Geometry check sheet. Reference: the model listing, model coordinates, mm. Face numbers are marked on the shaded views. A direction names the side the tool comes from. Round coordinates to 2 decimals unless told otherwise and drop trailing zeros. Write each loop counter-clockwise with the first axis right and the second up, starting at its lowest first coordinate (ties: lowest second). Pieces come first, ordered by that corner, then holes. Notation, with made-up numbers: M -4.75,62 L 16.25,62 A29 ccw 16.25,100 Z; hole C 26,21 d2. An arc over 180 degrees is marked long. Answer in a Markdown table with one row per item. Add a question column.
from build123d import *

# Parameters (mm, degrees)
BOSS_EXTRUDE1_DEPTH      = 10
BOSS_EXTRUDE1_DEPTH_BACK = 0.01
SKETCH3_W                = 37
SKETCH3_H                = 40
CUT_EXTRUDE1_DEPTH       = 3
SKETCH5_W                = 37
SKETCH5_H                = 40
CUT_EXTRUDE3_DEPTH       = 3
SKETCH7_W                = 165
SKETCH7_H                = 54
CUT_EXTRUDE4_DEPTH       = 6
SKETCH9_W                = 19
SKETCH9_H                = 16
SKETCH9_W_2              = 13.23867097
SKETCH9_H_2              = 10.64338859
SKETCH9_W_3              = 14.8958404
SKETCH9_H_3              = 14.23867097
BOSS_EXTRUDE2_DEPTH      = 20.3
SKETCH15_W               = 20
SKETCH15_H               = 50
BOSS_EXTRUDE3_DEPTH      = 20.3
SKETCH16_W               = 7.597238681
SKETCH16_H               = 8
SKETCH16_W_2             = 10
SKETCH16_H_2             = 9.4
SKETCH16_W_3             = 8.7
SKETCH16_H_3             = 8.5
SKETCH16_W_4             = 9.4
SKETCH16_H_4             = 9.3
BOSS_EXTRUDE4_DEPTH      = 30
SKETCH17_R               = 2.55
SKETCH17_R_2             = 3.5
CUT_EXTRUDE17_DEPTH      = 263.98121496
SKETCH18_W               = 43.4
SKETCH18_H               = 43.4
CUT_EXTRUDE18_DEPTH      = 3
SKETCH20_R               = 5
SKETCH20_R_2             = 4
CUT_EXTRUDE20_DEPTH      = 263.98121496
SKETCH21_R               = 9
CUT_EXTRUDE21_DEPTH      = 20
SKETCH22_R               = 1.55
CUT_EXTRUDE23_DEPTH      = 263.007861374
SKETCH25_W               = 7.9
SKETCH25_H               = 58.5
BOSS_EXTRUDE5_DEPTH      = 4
SKETCH26_W               = 7.816347336
SKETCH26_H               = 2.399791276
CUT_EXTRUDE24_DEPTH      = 58.5


with BuildPart() as part:
    # Sketch1 → Boss-Extrude1 (new, two sides: drawn at the far end of the back side and taken through both)
    with BuildSketch(Plane.XY.offset(-BOSS_EXTRUDE1_DEPTH_BACK)):
        with BuildLine():
            Line((0, 0), (0, -26))
            Line((0, -26), (60, -26))
            Line((60, -26), (60, -41))
            Line((60, -41), (33.129942315, -67.870057685))
            Line((33.129942315, -67.870057685), (-55.850057685, -67.870057685))
            ThreePointArc((-55.850057685, -67.870057685), (-169.745893523, -93.14097487), (-240, 0))
            ThreePointArc((-240, 0), (-169.745893523, 93.14097487), (-55.850057685, 67.870057685))
            Line((-55.850057685, 67.870057685), (33.129942315, 67.870057685))
            Line((33.129942315, 67.870057685), (60, 41))
            Line((60, 41), (60, 26))
            Line((60, 26), (0, 26))
            Line((0, 26), (0, 0))
        make_face()
    extrude(amount=BOSS_EXTRUDE1_DEPTH + BOSS_EXTRUDE1_DEPTH_BACK)

    # Sketch3 → Cut-Extrude1 (cut)
    with BuildSketch(Plane.XY.offset(10)):
        with Locations((-9.773002586, 47.870057685)):
            Rectangle(SKETCH3_W, SKETCH3_H)
    extrude(amount=-CUT_EXTRUDE1_DEPTH, mode=Mode.SUBTRACT)

    # Sketch5 → Cut-Extrude3 (cut)
    with BuildSketch(Plane.XY.offset(10)):
        with Locations((-9.773002586, -47.870057685)):
            Rectangle(SKETCH5_W, SKETCH5_H)
    extrude(amount=-CUT_EXTRUDE3_DEPTH, mode=Mode.SUBTRACT)

    # Sketch7 → Cut-Extrude4 (cut)
    with BuildSketch(Plane.XY.offset(10)):
        with Locations((-112.913094129, -21.943838981)):
            Rectangle(SKETCH7_W, SKETCH7_H)
    extrude(amount=-CUT_EXTRUDE4_DEPTH, mode=Mode.SUBTRACT)

    # Sketch9 → Boss-Extrude2 (add)
    with BuildSketch(Plane.XY.offset(10)):
        with Locations((-175.5, 33)):
            Rectangle(SKETCH9_W, SKETCH9_H)
        with Locations((-74.112324575, 12.332539195)):
            Rectangle(SKETCH9_W_2, SKETCH9_H_2)
        with Locations((-124.438795754, -58.044490005)):
            Rectangle(SKETCH9_W_3, SKETCH9_H_3)
    extrude(amount=BOSS_EXTRUDE2_DEPTH)

    # Sketch15 → Boss-Extrude3 (add)
    with BuildSketch(Plane.XY.offset(10)):
        with Locations((-10, 0.20156489)):
            Rectangle(SKETCH15_W, SKETCH15_H)
    extrude(amount=BOSS_EXTRUDE3_DEPTH)

    # Sketch16 → Boss-Extrude4 (add)
    with BuildSketch(Plane.XY.offset(10)):
        with Locations((-228.62215183, 0)):
            Rectangle(SKETCH16_W, SKETCH16_H)
        with Locations((-139.68812176, 89.3492876)):
            Rectangle(SKETCH16_W_2, SKETCH16_H_2)
        with Locations((-70.02791219, 66.09880262)):
            Rectangle(SKETCH16_W_3, SKETCH16_H_3)
        with Locations((-70.67791219, -66.2732878)):
            Rectangle(SKETCH16_W_4, SKETCH16_H_4)
        with Locations((-139.68812176, -88.33151307)):
            Rectangle(SKETCH16_W_2, SKETCH16_H_4)
    extrude(amount=BOSS_EXTRUDE4_DEPTH)

    # Sketch17 → Cut-Extrude17 (cut, through all)
    with BuildSketch(Plane.XY):
        with Locations((-228.42077117, 0)):
            Circle(SKETCH17_R)
        with Locations((-139.68812176, 89.6492876)):
            Circle(SKETCH17_R_2)
        with Locations((-69.87791219, 66.34880262)):
            Circle(SKETCH17_R_2)
        with Locations((-69.87791219, -66.6232878)):
            Circle(SKETCH17_R_2)
        with Locations((-139.68812176, -88.68151307)):
            Circle(SKETCH17_R_2)
    extrude(amount=CUT_EXTRUDE17_DEPTH, mode=Mode.SUBTRACT)

    # Sketch18 → Cut-Extrude18 (cut)
    with BuildSketch(Plane.XY.offset(10)):
        with Locations((-53.424548955, 39.3)):
            Rectangle(SKETCH18_W, SKETCH18_H)
    extrude(amount=-CUT_EXTRUDE18_DEPTH, mode=Mode.SUBTRACT)

    # Sketch20 → Cut-Extrude20 (cut, through all)
    with BuildSketch(Plane.XY):
        with Locations((-175.947050483, 32.112084796)):
            Circle(SKETCH20_R)
        with Locations((-124.709385772, -57.612858016)):
            Circle(SKETCH20_R)
        with Locations((-73.8879152, 12.75038661)):
            Circle(SKETCH20_R_2)
    extrude(amount=CUT_EXTRUDE20_DEPTH, mode=Mode.SUBTRACT)

    # Sketch21 → Cut-Extrude21 (cut)
    with BuildSketch(Plane(origin=(0, 0, 0), x_dir=(0, 0, -1), z_dir=(1, 0, 0))):
        with Locations((-19.36187505, 12.37175029)):
            Circle(SKETCH21_R)
        with Locations((-19.26539558, -14.62824971)):
            Circle(SKETCH21_R)
        with BuildLine():
            Line((-9.491579533, 2.276446619), (-9.557448357, -4.178698144))
            ThreePointArc((-9.557448357, -4.178698144), (-12.081396215, -6.651657156), (-14.554355227, -4.127709299))
            Line((-14.554355227, -4.127709299), (-14.488486403, 2.327435464))
            ThreePointArc((-14.488486403, 2.327435464), (-11.964538545, 4.800394476), (-9.491579533, 2.276446619))
        make_face()
    extrude(amount=-CUT_EXTRUDE21_DEPTH, mode=Mode.SUBTRACT)

    # Sketch22 → Cut-Extrude23 (cut, through all)
    with BuildSketch(Plane.XY.offset(7)):
        with Locations((-73.168620443, 58.97947337)):
            Circle(SKETCH22_R)
        with Locations((-33.768620443, 58.97947337)):
            Circle(SKETCH22_R)
        with Locations((-33.768620443, 19.57947337)):
            Circle(SKETCH22_R)
        with Locations((-73.168620443, 19.57947337)):
            Circle(SKETCH22_R)
    extrude(amount=-CUT_EXTRUDE23_DEPTH, mode=Mode.SUBTRACT)

    # Sketch25 → Boss-Extrude5 (add)
    with BuildSketch(Plane.XY.offset(10)):
        with Locations((-157.74640613, 41.59949177)):
            Rectangle(SKETCH25_W, SKETCH25_H)
    extrude(amount=BOSS_EXTRUDE5_DEPTH)

    # Sketch26 → Cut-Extrude24 (cut)
    with BuildSketch(Plane.XZ.offset(-12.34949177)):
        with Locations((-157.704579798, 11.208428435)):
            Rectangle(SKETCH26_W, SKETCH26_H)
    extrude(amount=-CUT_EXTRUDE24_DEPTH, mode=Mode.SUBTRACT)


solid = part.part
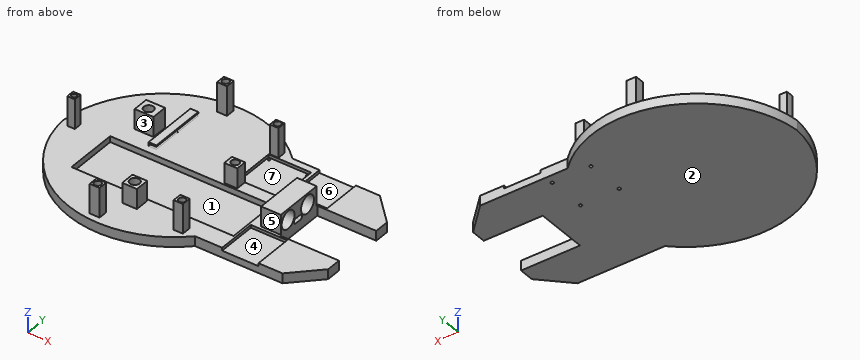
Item 1: Access from +Z, -Z, +X, -X, +Y, -Y to the whole of each face (thin tool, end or side, straight path). Record for the marked faces 1, 2, 3 and 4.
Item 2: Scan lines: probe 1 along X at (y, z) = (-1, 7.5); probe 2 along Z at (x, y) = (45.5, -50); probe 3 along Z at (x, y) = (-138.5, -46). Record each from-to range of solid material in increasing order. Write a range as from..to.
Item 3: Mould release check, pull along X, two halves, no side actions. Record for the marked faces 5, 6 and 7: +X half, -X half, draft (parallel to the pull), parting line (faces both ways), or undercut.
Item 4: Section check B-B, the plane x = -11. Record the boundary of the cut face in (y, z).
Item 5: Section check C-C, the plane x = -85.5. Record the boundary of the cut face in (y, z), and give its area (3 significant figures).
Item 6: Section check A-A, the plane z = 21.5. Give the number of separate pieces and of enclosed holes in the cut face, and give its area (3 significant figures).
Item 7: Gauge pin test, flat ends, axial feed: pin 1 Ø4 at (y, z) = (-49.5, 24.5) entering from -X; pin 2 Ø3 at (y, z) = (4.5, 9.5) entering from +X; pin 3 Ø6.5 at (x, y) = (-69.88, -66.62) entering from +Z. Record the tip position at first contact, or that the pin passes through.
Item 8: Section check D-D, the plane x = -125.5. Record the boundary of the cut face in (y, z), and give its area (3 significant figures).
Result sheet:
| question | item | result |
|---|---|---|
| 1 | face 1 | +Z |
| 1 | face 2 | -Z, +X, -X, +Y, -Y |
| 1 | face 3 | +Z, -X, -Y |
| 1 | face 4 | +Z, -Y |
| 2 | probe 1 | x = -239.92..-230.77, -226.08..-195.41, -30.41..0 |
| 2 | probe 2 | z = -0.01..10 |
| 2 | probe 3 | z = -0.01..4 |
| 3 | face 5 | draft |
| 3 | face 6 | undercut |
| 3 | face 7 | undercut |
| 4 | outline | M -67.87,-0.01 L 67.87,-0.01 L 67.87,7 L 27.87,7 L 27.87,10 L 25.2,10 L 25.2,30.3 L -24.8,30.3 L -24.8,10 L -27.87,10 L -27.87,7 L -67.87,7 Z; hole C -14.63,19.27 d18; hole M -4.18,9.56 L 2.28,9.49 A2.5 ccw 2.33,14.49 L -4.13,14.55 A2.5 ccw Z; hole C 12.37,19.36 d18 |
| 5 | outline | M -89.04,-0.01 L 89.04,-0.01 L 89.04,10 L 5.06,10 L 5.06,4 L -48.94,4 L -48.94,10 L -89.04,10 Z |
| 5 | area | 1,460 mm^2 |
| 6 | separate pieces | 11 |
| 6 | enclosed holes | 8 |
| 6 | area | 986 mm^2 |
| 7 | pin 1 | stops at x = -131.89 |
| 7 | pin 2 | stops at x = 0 |
| 7 | pin 3 | stops at z = 0 |
| 8 | outline | M -99.57,-0.01 L 99.57,-0.01 L 99.57,10 L 5.06,10 L 5.06,4 L -48.94,4 L -48.94,10 L -50.93,10 L -50.93,30.3 L -52.68,30.3 L -52.68,0 L -62.55,0 L -62.55,30.3 L -65.16,30.3 L -65.16,10 L -99.57,10 Z |
| 8 | area | 1,660 mm^2 |
